For this review, take the finished solid that the model builds, in its own axes (mm). Face numbers are marked on the shaded views. Give positions to 0.01 mm unless a question says otherwise; leave off trailing zeros. Order: outer loops, then holes, each group sorted by start corner. A loop starts at its lowest first (then second) coordinate and runs counter-clockwise, first axis right, second up. Notation, with made-up numbers: (-10, 79) -> (35, 79) arc R17 cw to (35, 98) -> close; hole circle Ø10 at (80.25, 16.5). An arc over 180 degrees is marked (long way). Use CSV: the item, a comma, the result in double quotes. Start each with the question number.
```python
from build123d import *

# Parameters (mm, degrees)
F0_R     = 3.175
F1_DEPTH = 12.7
F2_R     = 5.08
F3_DEPTH = 3.81


# Not quite as in the source:
# - a fillet or chamfer that OpenCascade refuses, or shapes differently, is made with other operations: its cross-section is extruded or revolved along the edge and cut away or added


with BuildPart() as f1:
    # F0 (on Top) → F1 (new body)
    with BuildSketch(Plane.XY):
        with Locations((-67.7428916097, -29.48333323)):
            Circle(F0_R)
    extrude(amount=F1_DEPTH)

    # F2 (on face) → F3 (join)
    with BuildSketch(Plane.XY.offset(12.7)):
        with Locations((-67.7428916097, -29.48333323)):
            Circle(F2_R)
    extrude(amount=F3_DEPTH)

    # F4: fillet of radius 5.08 on 1 edges, made by hand

    # F4_s1 → F4_t2 (revolve, cut)
    with BuildSketch(Plane.XZ.offset(29.48333323)):
        with BuildLine():
            ThreePointArc((-62.6628916097, 12.7), (-64.470728486, 15.4460926284), (-67.5815804594, 16.51))
            Line((-67.5815804594, 16.51), (-62.6628916097, 16.51))
            Line((-62.6628916097, 16.51), (-62.6628916097, 12.7))
        make_face()
    revolve(axis=Axis((-67.7428916097, -29.48333323, 16.51), (0, 0, 1)), mode=Mode.SUBTRACT)


solid = f1.part
```
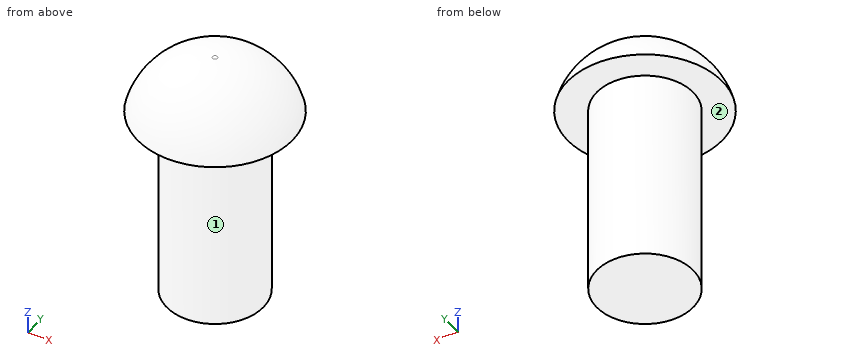
1. Consider section A-A (z = 2.25). State the section outline as (x, y) points (3 decimals).
2. To check wall thickness, follow L1, parallel to X at y = -29.5, z = 10; L2, parallel to X at y = -27.5, z = 3.5; L3, parallel to Z at x = -67.5, y = -34. State the ranges of each line that lie inside material, in increasing order. Write a range as [from, to].
3. Draft analysis for pull direction Y (two halves, no side actions). For the marked faces 1 and 2, state which applies: +Y half, -Y half, draft (parallel to the pull), parting line (faces both ways), or undercut.
4. Clearance check with flat-ended pins moving along their axes: P1, Ø1, axis at x = -65, y = -30.5, coming from the +Z side; P2, Ø1.5, axis at y = -32.5, z = 5.5, coming from the +X side; P3, Ø6, axis at x = -67, z = 4, coming from the -Y side. State where each tip first meets the part, or that it passes through.
Answer list:
1,outline,"circle Ø6.35 at (-67.743, -29.483)"
2,L1,"[-70.92, -64.57]"
2,L2,"[-70.22, -65.26]"
2,L3,"[12.7, 14.03]"
3,face 1,"parting line"
3,face 2,"draft"
4,P1,"z = 15.98"
4,P2,"x = -65.52"
4,P3,"y = -32.66"
